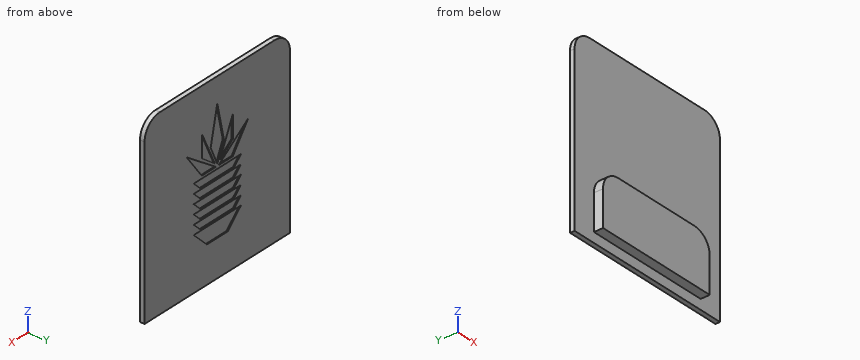
from build123d import *

# Parameters (mm, degrees)
SKETCH1_W           = 120.65
SKETCH1_H           = 127
BOSS_EXTRUDE1_DEPTH = 3.175
FILLET1_R           = 12.7
BOSS_EXTRUDE2_DEPTH = 6.35
CUT_EXTRUDE1_START  = -0.79375
CUT_EXTRUDE1_DEPTH  = 0.79375


# Read off the part's stored shape, not the designer's step: Cut-Extrude1
with BuildPart() as part:
    # Sketch1 → Boss-Extrude1 (new body)
    with BuildSketch(Plane(origin=(0, 0, 0), x_dir=(1, 0, 0), z_dir=(0, 1, 0))):
        Rectangle(SKETCH1_W, SKETCH1_H)
    extrude(amount=BOSS_EXTRUDE1_DEPTH)

    # Fillet1
    fillet1_edges = [part.edges().sort_by_distance(p)[0] for p in [
        (60.325, 1.5875, 63.5),
        (-60.325, 1.5875, 63.5),
    ]]
    fillet(fillet1_edges, radius=FILLET1_R)

    # Sketch2 → Boss-Extrude2 (add)
    with BuildSketch(Plane.XZ):
        with BuildLine():
            Line((-44.2595, -32.004), (-44.2595, -56.642))
            Line((-44.2595, -56.642), (44.2595, -56.642))
            Line((44.2595, -56.642), (44.2595, -32.004))
            ThreePointArc((44.2595, -32.004), (40.539756121, -23.023743879), (31.5595, -19.304))
            Line((31.5595, -19.304), (-31.5595, -19.304))
            ThreePointArc((-31.5595, -19.304), (-40.539756121, -23.023743879), (-44.2595, -32.004))
        make_face()
    extrude(amount=BOSS_EXTRUDE2_DEPTH)

    # Cut-Extrude1 outline → Cut-Extrude1 (cut)
    with BuildSketch(Plane(origin=(0, 3.175, 0), x_dir=(1, 0, 0), z_dir=(0, 1, 0)).offset(CUT_EXTRUDE1_START)):
        Polygon((19.586934791, 20.568683014), (13.900914294, 26.330878533), (-13.900917809, 26.330878533), (-19.586938306, 20.568683014), align=None)
        Polygon((25.558154067, -24.714180755), (12.840680417, -7.047287084), (1.136138921, -7.047287084), align=None)
        Polygon((-25.558126027, -24.714180755), (-1.13611088, -7.047287084), (-12.840652376, -7.047287084), align=None)
        Polygon((12.872252496, -17.941870118), (1.967957375, -9.461750192), (12.872252496, -33.488756649), align=None)
        Polygon((19.586934791, 14.109110528), (13.900914294, 19.871337603), (-13.900917809, 19.871337603), (-19.586938306, 14.109110528), align=None)
        Polygon((19.586934791, 7.649569598), (13.900882739, 13.411796673), (-13.900886254, 13.411796673), (-19.586938306, 7.649569598), align=None)
        Polygon((19.586934791, 1.190028667), (13.900914294, 6.952224187), (-13.900917809, 6.952224187), (-19.586938306, 1.190028667), align=None)
        Polygon((19.586934791, -5.269543818), (13.900914294, 0.492683256), (-13.900917809, 0.492683256), (-19.586938306, -5.269543818), align=None)
        Polygon((0, -8.460639301), (-5.496493939, -21.106287094), (0, -46.231527771), (5.496493939, -21.106287094), align=None)
        Polygon((-1.967957374, -9.461750193), (-12.872252495, -17.941870118), (-12.872252495, -33.488756649), align=None)
        Polygon((8.661555888, 38.1), (-8.661555888, 38.1), (-19.58692752, 27.028231496), (19.58692752, 27.028231496), align=None)
    extrude(amount=CUT_EXTRUDE1_DEPTH, mode=Mode.SUBTRACT)


solid = part.part
Check sheet for the modelled part. Datum: model origin and axes. Units: mm. Round coordinates to 2 decimals unless told otherwise and drop trailing zeros. Order: outer loops, then holes, each group sorted by start corner. A loop starts at its lowest first (then second) coordinate and runs counter-clockwise, first axis right, second up.
(1) Go/stop test with flat-tipped pins: P1, Ø1.7, axis at x = -0.5, z = -22.5, coming from the +Y side; P2, Ø6.5, axis at x = 8, z = -3.5, coming from the +Y side (3 decimals); P3, Ø2, axis at x = 48, y = -2.5, coming from the -Z side; P4, Ø4, axis at x = 25, y = -2.5, coming from the -Z side. Record where each tip stops, or that it passes through.
(2) Cross-section at B-B, the plane y = -3.75. Enter the section's corners in (x, z).
(3) Cross-section at C-C, the plane x = 38. Enter the section's corners in (y, z) (3 decimals), and give its area (3 significant figures).
(4) Cross-section at D-D, the plane z = -22. Enter the section's corners in (x, y) (3 decimals).
(5) Scan lines: probe 1 along Y at (x, z) = (-51.5, 49) (3 decimals); probe 2 along Z at (x, y) = (-22, -4.25); probe 3 along Z at (x, y) = (-40.5, -2.75). Record each from-to range of solid material in increasing order.
Check sheet entries:
1. P1: stops at y = 2.38
1. P2: stops at y = 3.175
1. P3: passes through
1. P4: stops at z = -56.64
2. outline: (-44.26, -56.64) - (44.26, -56.64) - (44.26, -32) arc R12.7 ccw to (31.56, -19.3) - (-31.56, -19.3) arc R12.7 ccw to (-44.26, -32) - close
3. outline: (-6.35, -56.642) - (0, -56.642) - (0, -63.5) - (3.175, -63.5) - (3.175, 63.5) - (0, 63.5) - (0, -21.058) - (-6.35, -21.058) - close
3. area: 629 mm2
4. outline: (-60.325, 0) - (-39.383, 0) - (-39.383, -6.35) - (39.383, -6.35) - (39.383, 0) - (60.325, 0) - (60.325, 3.175) - (18.175, 3.175) - (18.175, 2.381) - (-18.175, 2.381) - (-18.175, 3.175) - (-60.325, 3.175) - close
5. probe 1: y = 0 to 3.175
5. probe 2: z = -56.64 to -19.3
5. probe 3: z = -56.64 to -22.98
